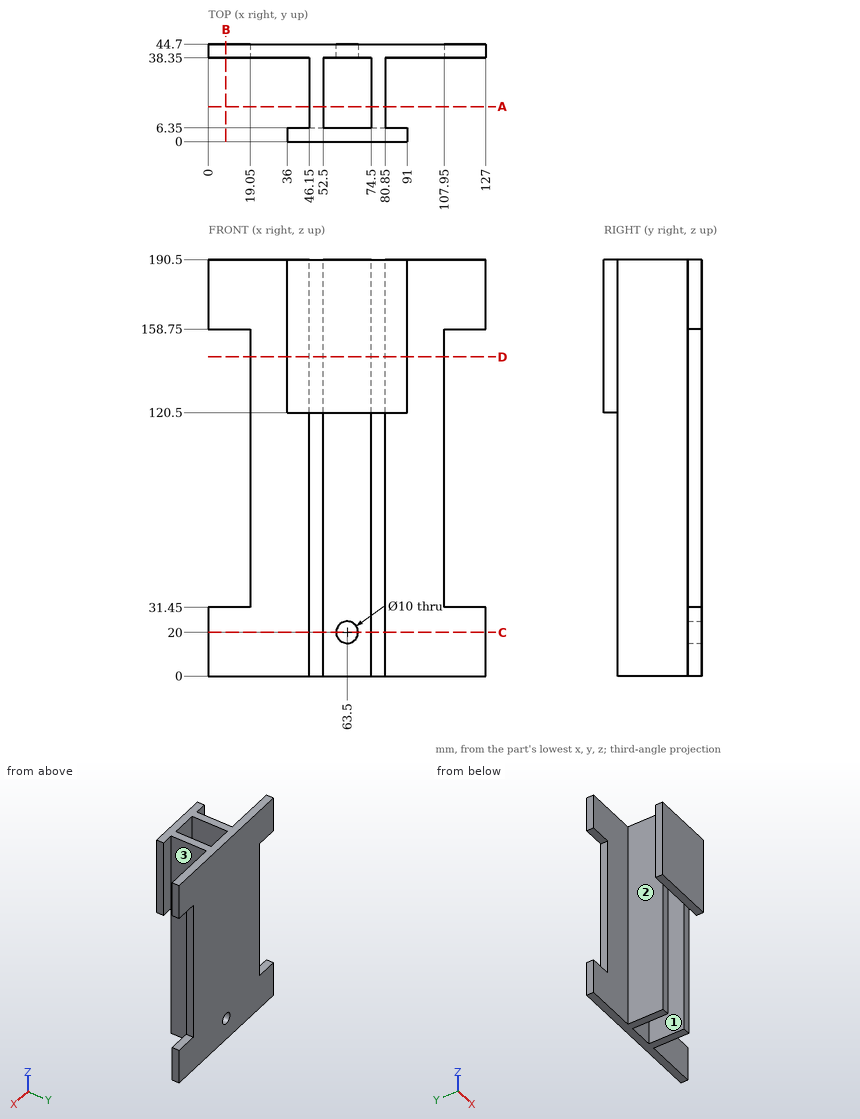
Verification items for this drawing (mm, ordinates from the low corner). A direction names the side the tool comes from. Give positions to 0.01 mm unless a question says otherwise; leave off trailing zeros. Write each loop counter-clockwise with the first axis right and the second up, starting at its lowest first coordinate (ties: lowest second). Pieces come first, ordered by that corner, then holes. Notation, with made-up numbers: (-8, -11.5) -> (9, -11.5) arc R10 ccw to (9, -6.5) -> close; hole circle Ø5 at (48.5, 71). An arc over 180 degrees is marked (long way). Use CSV: the item, a comma, the result in double quotes. Start each with the question number.
Q1. Tool access check on the marked faces 1, 2 and 3. Record the directions out of +Z, -Z, +X, -X, +Y, -Y that give a thin tool (end or side, any length) a straight path to the whole face; none if there is none.
Q2. Scan lines: line 1 along Z through (x, y) = (63, 40); line 2 along X through (y, z) = (26, 105.5); line 3 along Y through (x, z) = (21.5, 98.5). Record each from-to range of solid material in increasing order.
Q3. Cross-section at B-B on x = 8. Enter the section's corners in (y, z), and give its area (3 significant figures).
Q4. Depth check by flat-ended pin: P1, Ø10, axis at y = 28.5, z = 98, coming from the -X side; P2, Ø1, axis at y = 5, z = 155.5, coming from the +X side; P3, Ø1.9, axis at y = 43, z = 93, coming from the +X side; P4, Ø9, axis at x = 63.5, z = 20, coming from the +Y side. Enter the tip coordinate at first touch or a pass-through.
Q5. Cross-section at C-C on z = 20. Enter the section's corners in (x, y), and give its area (3 significant figures).
Q6. Cross-section at D-D on z = 146. Enter the section's corners in (x, y), and give its area (3 significant figures).
Q7. Cross-section at A-A on y = 16. Enter the section's corners in (x, z), and give its area (3 significant figures).
Working result:
1,face 1,"+Z, -Z"
1,face 2,"+Z, -Z, -X"
1,face 3,"+Z, -Z, +X"
2,line 1,"z = 0 to 15.03, 24.97 to 190.5"
2,line 2,"x = 46.15 to 52.5, 74.5 to 80.85"
2,line 3,"y = 38.35 to 44.7"
3,outline,"(38.35, 0) -> (44.7, 0) -> (44.7, 31.45) -> (38.35, 31.45) -> close; (38.35, 158.75) -> (44.7, 158.75) -> (44.7, 190.5) -> (38.35, 190.5) -> close"
3,area,"401 mm^2"
4,P1,"stops at x = 46.15"
4,P2,"stops at x = 91"
4,P3,"stops at x = 107.95"
4,P4,"passes through"
5,outline,"(0, 38.35) -> (46.15, 38.35) -> (46.15, 6.35) -> (52.5, 6.35) -> (52.5, 38.35) -> (58.5, 38.35) -> (58.5, 44.7) -> (0, 44.7) -> close; (68.5, 38.35) -> (74.5, 38.35) -> (74.5, 6.35) -> (80.85, 6.35) -> (80.85, 38.35) -> (127, 38.35) -> (127, 44.7) -> (68.5, 44.7) -> close"
5,area,"1,150 mm^2"
6,outline,"(19.05, 38.35) -> (46.15, 38.35) -> (46.15, 6.35) -> (36, 6.35) -> (36, 0) -> (91, 0) -> (91, 6.35) -> (80.85, 6.35) -> (80.85, 38.35) -> (107.95, 38.35) -> (107.95, 44.7) -> (19.05, 44.7) -> close; hole (52.5, 6.35) -> (74.5, 6.35) -> (74.5, 38.35) -> (52.5, 38.35) -> close"
6,area,"1,320 mm^2"
7,outline,"(46.15, 0) -> (52.5, 0) -> (52.5, 190.5) -> (46.15, 190.5) -> close; (74.5, 0) -> (80.85, 0) -> (80.85, 190.5) -> (74.5, 190.5) -> close"
7,area,"2,420 mm^2"
